from build123d import *

# Parameters (mm, degrees)
SKETCH1_W            = 78
SKETCH1_H            = 92.5
SKETCH1_R            = 1.4
SKETCH1_R_2          = 3.5
SKETCH1_W_2          = 6
SKETCH1_H_2          = 50
SKETCH1_W_3          = 3.5
SKETCH1_H_3          = 6
SKETCH1_H_4          = 49.3
SKETCH1_H_5          = 41
SKETCH1_H_6          = 11.5
SKETCH1_H_7          = 3.5
SKETCH1_W_4          = 8.5
BASE_DEPTH           = 10
SKETCH2_W            = 71.5
SKETCH2_H            = 84
PCB_CUTOUT_DEPTH     = 6
SKETCH3_W            = 9
SKETCH3_H            = 6.6
USB_SLOT_DEPTH       = 4.25
F_1MM_EDGE_FILLETS_R = 1


with BuildPart() as part:
    # Sketch1 → Base (new body)
    with BuildSketch(Plane(origin=(0, 0, 0), x_dir=(1, 0, 0), z_dir=(0, 1, 0))):
        Rectangle(SKETCH1_W, SKETCH1_H)
        with Locations(Location((-24.13, 12.05, 0), (0, 0, 270))):
            Circle(SKETCH1_R, mode=Mode.SUBTRACT)
        with Locations(Location((24.13, 13.32, 0), (0, 0, 270))):
            Circle(SKETCH1_R, mode=Mode.SUBTRACT)
        with Locations(Location((-8.89, -38.75, 0), (0, 0, 270))):
            Circle(SKETCH1_R, mode=Mode.SUBTRACT)
        with Locations(Location((8.2055, 12.0071, 0), (0, 0, 270))):
            Circle(SKETCH1_R_2, mode=Mode.SUBTRACT)
        with Locations(Location((-8.3159, 12.0071, 0), (0, 0, 270))):
            Circle(SKETCH1_R_2, mode=Mode.SUBTRACT)
        with Locations((-30.5, -13.5)):
            Rectangle(SKETCH1_W_2, SKETCH1_H_2, mode=Mode.SUBTRACT)
        with Locations((30.5, -13.5)):
            Rectangle(SKETCH1_W_2, SKETCH1_H_2, mode=Mode.SUBTRACT)
        with Locations((31.75, 36.25)):
            Rectangle(SKETCH1_W_3, SKETCH1_H_3, mode=Mode.SUBTRACT)
        with Locations((-31.75, 36.25)):
            Rectangle(SKETCH1_W_3, SKETCH1_H_3, mode=Mode.SUBTRACT)
        Polygon((25, 34.25), (25, 23.75), (19.5, 23.75), (19.5, 16.75), (25, 16.75), (25, 17.75), (28.5, 17.75), (28.5, 34.25), align=None, mode=Mode.SUBTRACT)
        with Locations((-24.15, -14.15)):
            Rectangle(SKETCH1_W_3, SKETCH1_H_4, mode=Mode.SUBTRACT)
        with Locations((24.15, -18.3)):
            Rectangle(SKETCH1_W_3, SKETCH1_H_5, mode=Mode.SUBTRACT)
        with Locations((12.75, 34.75)):
            Rectangle(SKETCH1_W_3, SKETCH1_H_6, mode=Mode.SUBTRACT)
        with Locations((0.5, 38.75)):
            Rectangle(SKETCH1_W_2, SKETCH1_H_7, mode=Mode.SUBTRACT)
        with Locations((-10.88, 6.3)):
            Rectangle(SKETCH1_W_4, SKETCH1_H_7, mode=Mode.SUBTRACT)
        with Locations((0.62, 0)):
            Rectangle(SKETCH1_W_2, SKETCH1_H_7, mode=Mode.SUBTRACT)
    extrude(amount=BASE_DEPTH)

    # Sketch2 → PCB Cutout (cut)
    with BuildSketch(Plane.XZ.offset(-10)):
        Rectangle(SKETCH2_W, SKETCH2_H)
    extrude(amount=PCB_CUTOUT_DEPTH, mode=Mode.SUBTRACT)

    # Sketch3 → USB Slot (cut)
    with BuildSketch(Plane(origin=(0, 0, -46.25), x_dir=(-1, 0, 0), z_dir=(0, 0, -1))):
        with Locations((11.9, 6.7)):
            Rectangle(SKETCH3_W, SKETCH3_H)
    extrude(amount=-USB_SLOT_DEPTH, mode=Mode.SUBTRACT)

    # 1mm Edge Fillets
    f_1mm_edge_fillets_edges = [part.edges().sort_by_distance(p)[0] for p in [
        (0, 0, -46.25),
        (39, 0, 0),
        (0, 0, 46.25),
        (-39, 0, 0),
        (-39, 5, -46.25),
        (39, 5, -46.25),
        (39, 5, 46.25),
        (-39, 5, 46.25),
    ]]
    fillet(f_1mm_edge_fillets_edges, radius=F_1MM_EDGE_FILLETS_R)


solid = part.part
The listing builds one solid part. Answer for the finished solid, in the listing's coordinates (mm). A direction names the side the tool comes from. Coordinates: 2 decimals unless noted, no trailing zeros. Loops run counter-clockwise (first coordinate to the right, second up) from the corner with the lowest first, then second, coordinate; pieces in that order, holes last. Notation, with made-up numbers: (51.5, -21.5) -> (82.5, -21.5) arc R14 ccw to (82.5, -3.5) -> close; hole circle Ø9 at (13, 85.25). An arc over 180 degrees is marked (long way). Answer in a Markdown table with one row per item. Add a question column.
1. For faces 4 (the flat face through (-26, 7, -42)), 5 (the flat face through (-7.4, 7, -44)), 6 (the flat face through (27, 2, -34.25)), determine the directions among +Z, -Z, +X, -X, +Y, -Y from which every point of the face is accessible in a straight line to the end or side of a thin tool.
2. The part is cut by section B-B, the plane x = -24.13. Write down the section's boundary in (y, z).
3. Flat-ended cylindrical pins translate along their axes: P1, Ø8, axis at x = -11, z = -10.5, coming from the -Y side; P2, Ø4, axis at x = 3.5, z = -8.5, coming from the +Y side. Find the tip coordinate at first contact, or state that the pin passes through.
4. The part is cut by section C-C, the plane y = 6.25. Write down the section's boundary in (x, z), then the cut area to 3 significant figures.
5. Determine the mould class of faces 1 (the flat face through (39, 5, 1)), 2 (the cylindrical face through (-7.26, 1.97, -8.67)), 3 (the flat face through (-1, 5, -46.25)) for opening direction X: +X half, -X half, draft (parallel to the pull), parting line (faces both ways), or undercut.
6. Consider line 1 (Z direction, x = -0.5, y = 1.25); line 2 (X direction, y = 5.5, z = -18.5); line 3 (X direction, y = 2.9, z = 38.75). Determine where each line is inside the solid, lowest interval first. Write a range as [from, to].
7. The part is cut by section A-A, the plane z = 24.5. Write down the section's boundary in (x, y).
Answer below:
| question | item | result |
|---|---|---|
| 1 | face 4 | +Y |
| 1 | face 5 | -Z, +Y |
| 1 | face 6 | +Y, -Y |
| 2 | outline | (0, -45.25) arc R1 ccw to (1, -46.25) -> (10, -46.25) -> (10, -42) -> (4, -42) -> (4, -13.45) -> (0, -13.45) -> close; (0, -10.65) -> (4, -10.65) -> (4, -10.5) -> (0, -10.5) -> close; (0, 38.8) -> (4, 38.8) -> (4, 42) -> (10, 42) -> (10, 46.25) -> (1, 46.25) arc R1 ccw to (0, 45.25) -> close |
| 3 | P1 | y = 0 |
| 3 | P2 | y = 4 |
| 4 | outline | (-39, -45.25) arc R1 ccw to (-38, -46.25) -> (-16.4, -46.25) -> (-16.4, -42) -> (-35.75, -42) -> (-35.75, 42) -> (35.75, 42) -> (35.75, -42) -> (-7.4, -42) -> (-7.4, -46.25) -> (38, -46.25) arc R1 ccw to (39, -45.25) -> (39, 45.25) arc R1 ccw to (38, 46.25) -> (-38, 46.25) arc R1 ccw to (-39, 45.25) -> close |
| 4 | area | 1,170 mm2 |
| 5 | face 1 | +X half |
| 5 | face 2 | undercut |
| 5 | face 3 | draft |
| 6 | line 1 | [-46.25, -40.5], [-37, -1.75], [1.75, 46.25] |
| 6 | line 2 | [-39, -35.75], [35.75, 39] |
| 6 | line 3 | [-39, -25.9], [-22.4, -10.29], [-7.49, 22.4], [25.9, 39] |
| 7 | outline | (-39, 1) arc R1 ccw to (-38, 0) -> (-33.5, 0) -> (-33.5, 4) -> (-35.75, 4) -> (-35.75, 10) -> (-39, 10) -> close; (-27.5, 0) -> (-25.9, 0) -> (-25.9, 4) -> (-27.5, 4) -> close; (-22.4, 0) -> (22.4, 0) -> (22.4, 4) -> (-22.4, 4) -> close; (25.9, 0) -> (27.5, 0) -> (27.5, 4) -> (25.9, 4) -> close; (33.5, 0) -> (38, 0) arc R1 ccw to (39, 1) -> (39, 10) -> (35.75, 10) -> (35.75, 4) -> (33.5, 4) -> close |
